Build history of the part. All positions in model axes, mm. A direction names the side the tool comes from. Coordinates: 2 decimals unless noted, no trailing zeros. Write each loop counter-clockwise with the first axis right and the second up, starting at its lowest first coordinate (ties: lowest second). Pieces come first, ordered by that corner, then holes.
```python
from build123d import *

# Parameters (mm, degrees)
BOSS_EXTRUDE1_DEPTH = 228.6
SKETCH3_R           = 2.413
CUT_EXTRUDE1_DEPTH  = 1.905
LPATTERN1_COUNT     = 3
LPATTERN1_PITCH     = 76.2
SKETCH4_W           = 22.804701919
SKETCH4_H           = 24.737303777
CUT_EXTRUDE2_DEPTH  = 342.9


with BuildPart() as part:
    # Sketch2 → Boss-Extrude1 (new, symmetric)
    with BuildSketch(Plane(origin=(0, 0, 0), x_dir=(0, 0, -1), z_dir=(1, 0, 0))):
        Polygon((0, 9.144), (-12.192, 9.144), (-12.192, 4.445), (-10.6045, 4.445), (-10.6045, 5.969), (-4.2545, 5.969), (-4.2545, 4.445), (-1.905, 4.445), (-1.905, -4.445), (-4.2545, -4.445), (-4.2545, -5.969), (-10.6045, -5.969), (-10.6045, -4.445), (-12.192, -4.445), (-12.192, -9.144), (0, -9.144), align=None)
    extrude(amount=BOSS_EXTRUDE1_DEPTH, both=True)

    # Sketch3 → Cut-Extrude1 (cut)
    with BuildSketch(Plane.XY.offset(1.905)):
        with Locations((38.1, 0)):
            Circle(SKETCH3_R)
    cut_extrude1 = extrude(amount=-CUT_EXTRUDE1_DEPTH, mode=Mode.SUBTRACT)

    # LPattern1: Cut-Extrude1 ×3
    with Locations(*[(i * LPATTERN1_PITCH, 0, 0) for i in range(1, LPATTERN1_COUNT)]):
        add(cut_extrude1, mode=Mode.SUBTRACT)

    # SurfaceCut1
    split(bisect_by=Plane(origin=(0, 0, 0), x_dir=(0, 0, -1), z_dir=(1, 0, 0)), keep=Keep.TOP)

    # Mirror1: part across plane


with BuildPart() as part_1:
    add(part.part)
    add(part.part.mirror(Plane(origin=(0, 0, 0), x_dir=(0, 0, 1), z_dir=(1, 0, 0))))

    # Sketch4 → Cut-Extrude2 (cut)
    with BuildSketch(Plane(origin=(228.6, 0, 0), x_dir=(0, 0, -1), z_dir=(1, 0, 0))):
        with Locations((-5.709479629, -0.367194353)):
            Rectangle(SKETCH4_W, SKETCH4_H)
    extrude(amount=-CUT_EXTRUDE2_DEPTH, mode=Mode.SUBTRACT)


solid = part_1.part
```
1. Saw through at A-A on y = 0. List the corners of the cut face in (x, z) (3 decimals).
Computed values:
outline: (-228.6, 0) - (-192.913, 0) - (-192.913, 1.905) - (-228.6, 1.905) - close; (-188.087, 0) - (-116.713, 0) - (-116.713, 1.905) - (-188.087, 1.905) - close
2. Saw through at C-C on x = -190.5. List the corners of the cut face in (y, z) (1 decimal), plus the area to 3 significant figures.
Computed values:
outline: (-9.1, 0) - (-2.4, 0) - (-2.4, 1.9) - (-4.4, 1.9) - (-4.4, 4.3) - (-6, 4.3) - (-6, 10.6) - (-4.4, 10.6) - (-4.4, 12.2) - (-9.1, 12.2) - close; (2.4, 0) - (9.1, 0) - (9.1, 12.2) - (4.4, 12.2) - (4.4, 10.6) - (6, 10.6) - (6, 4.3) - (4.4, 4.3) - (4.4, 1.9) - (2.4, 1.9) - close
area: 103 mm2
3. Saw through at D-D on x = -207.5. List the corners of the cut face in (y, z) (1 decimal), plus the area to 3 significant figures.
Computed values:
outline: (-9.1, 0) - (9.1, 0) - (9.1, 12.2) - (4.4, 12.2) - (4.4, 10.6) - (6, 10.6) - (6, 4.3) - (4.4, 4.3) - (4.4, 1.9) - (-4.4, 1.9) - (-4.4, 4.3) - (-6, 4.3) - (-6, 10.6) - (-4.4, 10.6) - (-4.4, 12.2) - (-9.1, 12.2) - close
area: 112 mm2
4. Mould opens along Y. For faces 4 (the face through (-116.712, -0.053, 0.966)), 5 (the face through (-172, 9.144, 6)), 6 (the face through (-172, 0, 0)), 7 (the face through (-172, -4.445, 3)) say: +Y half, -Y half, draft (parallel to the pull), parting line (faces both ways), or undercut.
Computed values:
face 4: undercut
face 5: +Y half
face 6: draft
face 7: undercut
5. Probe line 1 along Y through (x, z) = (-190.5, 1.2); line 2 along Y through (x, z) = (-213, 10.25); line 3 along Z through (x, y) = (-123, 4.75). List the from-to ranges inside material, lowest first.
Computed values:
line 1: y = -9.14 to -2.41, 2.41 to 9.14
line 2: y = -9.14 to -5.97, 5.97 to 9.14
line 3: z = 0 to 4.25, 10.6 to 12.19
6. Saw through at B-B on z = 8. List the corners of the cut face in (x, y).
Computed values:
outline: (-228.6, -9.14) - (-114.3, -9.14) - (-114.3, -5.97) - (-228.6, -5.97) - close; (-228.6, 5.97) - (-114.3, 5.97) - (-114.3, 9.14) - (-228.6, 9.14) - close
7. Flat gauge pin, fed straight in: pin 1 (4.5 mm diameter, centred on x = -180, y = 1, fed in from +Z) (3 decimals). Where does the tip first touch, or does it go through?
Computed values:
pin 1: stops at z = 1.905
8. 3-axis set-ups, long thin cutter, end or side, ignore diameter. For faces 1 (the face through (-172, 0, 1.905)), 2 (the face through (-114.3, 7, 6)), 3 (the face through (-172, 5.969, 7)): which of +Z, -Z, +X, -X, +Y, -Y reach the whole face in a straight line?
Computed values:
face 1: +Z, +X, -X
face 2: +Z, -Z, +X, +Y, -Y
face 3: +X, -X
